from build123d import *

# Parameters (mm, degrees)
CYLINDER002_R     = 2
CYLINDER002_DEPTH = 22
CYLINDER001_R     = 9
CYLINDER001_DEPTH = 1120
CYLINDER_R        = 11
CYLINDER_DEPTH    = 1120


with BuildPart() as cylinder002:
    # Cylinder002 → Cylinder002 (new body)
    with BuildSketch(Plane(origin=(-11, 0, 0), x_dir=(0, 0, -1), z_dir=(1, 0, 0))):
        Circle(CYLINDER002_R)
    extrude(amount=CYLINDER002_DEPTH)


with BuildPart() as cylinder001:
    # Cylinder001 → Cylinder001 (new body)
    with BuildSketch(Plane.XY):
        Circle(CYLINDER001_R)
    extrude(amount=CYLINDER001_DEPTH)


with BuildPart() as body:
    # Cylinder → Cylinder (new body)
    with BuildSketch(Plane.XY):
        Circle(CYLINDER_R)
    extrude(amount=CYLINDER_DEPTH)

    # Cut: cut Cylinder001
    add(cylinder001.part, mode=Mode.SUBTRACT)

    # Cut001: cut Cylinder002
    add(cylinder002.part, mode=Mode.SUBTRACT)


solid = body.part
Source: CAD feature listing. Evaluate the final solid. Frame: model axes, mm. Round coordinates to 2 decimals unless told otherwise and drop trailing zeros. Write each loop counter-clockwise with the first axis right and the second up, starting at its lowest first coordinate (ties: lowest second). Pieces come first, ordered by that corner, then holes. Notation, with made-up numbers: (84.5, 88) - (125.5, 88) arc R5 cw to (125.5, 94) - close; hole circle Ø10 at (59, 66.25). An arc over 180 degrees is marked (long way). Use CSV: the item, a comma, the result in double quotes. Start each with the question number.
(1) Material intervals for probe 1 along X at (y, z) = (-1.5, 518.5); probe 2 along Y at (x, z) = (2.5, 537); probe 3 along X at (y, z) = (0, 574.5), sorted ascending. Write a range as [from, to].
(2) First-contact query: pin 1 Ø6 at (x, y) = (-2.5, -2.5) entering from +Z; pin 2 Ø3 at (x, z) = (-2, 870.5) entering from +Y; pin 3 Ø6 at (x, z) = (8, 311) entering from +Y; pin 4 Ø1 at (y, z) = (-1, 874) entering from -X. Flat tips, straight axial feed; report the tip coordinate or a pass-through.
(3) Cut plane A-A, the plane x = 0. Return loops of the section in (y, z), and give its area (3 significant figures).
(4) Mould query, pull axis Y, two halves, no side actions, for faces 1 (the face through (2, -9, 1120)), 2 (the face through (-2.38, -10.74, 552.16)), 3 (the face through (-1.172, 8.923, 552.16)). Classes: pulls with the +Y half, pulls with the -Y half, needs draft (parallel to the pull), parting line crosses it, or undercut.
(5) Cut plane B-B, the plane z = 764.5. Return loops of the section in (x, y), and give its area (3 significant figures).
Geometry says:
1,probe 1,"[-10.9, -8.87], [8.87, 10.9]"
1,probe 2,"[-10.71, -8.65], [8.65, 10.71]"
1,probe 3,"[-11, -9], [9, 11]"
2,pin 1,"through"
2,pin 2,"y = 10.99"
2,pin 3,"y = 9.8"
2,pin 4,"x = -10.99"
3,outline,"(-11, 0) - (-9, 0) - (-9, 1120) - (-11, 1120) - close; (9, 0) - (11, 0) - (11, 1120) - (9, 1120) - close"
3,area,"4,480 mm²"
4,face 1,"needs draft"
4,face 2,"parting line crosses it"
4,face 3,"undercut"
5,outline,"circle Ø22 at (0, 0); hole circle Ø18 at (0, 0)"
5,area,"126 mm²"
